Verification items for this drawing (mm, ordinates from the low corner). A direction names the side the tool comes from. Coordinates: 2 decimals unless noted, no trailing zeros. Write each loop counter-clockwise with the first axis right and the second up, starting at its lowest first coordinate (ties: lowest second). Pieces come first, ordered by that corner, then holes. Notation, with made-up numbers: (-35, 82.25) -> (14, 82.25) arc R19 ccw to (14, 119.25) -> close; hole circle Ø6 at (37, 82). An arc over 180 degrees is marked (long way). One line per item, written item: value. Start each with the question number.
1) Draft check along X on the marked faces 1, 2 and 3. Enter one of: +X half, -X half, draft (parallel to the pull), parting line (faces both ways), or undercut.
2) Scan lines: line 1 along Y through (x, z) = (3.5, 17.25); line 2 along Z through (x, y) = (5.25, 0.55); line 3 along Y through (x, z) = (2.5, 17.5). Record each from-to range of solid material in increasing order. Write a range as [from, to].
3) Sectioned sample at C-C on y = 0.5. Enter the section's corners in (x, z) (1 decimal), plus the area to 3 significant figures.
4) Sectioned sample at A-A on x = 5.5. Enter the section's corners in (y, z), plus the area to 3 significant figures.
5) Set-up check for the marked faces 4 and 5: record each of +Z, -Z, +X, -X, +Y, -Y from which the full face is reachable in a straight line by a thin tool's end or side.
6) Gauge pin test, flat ends, axial feed: P1, Ø3, axis at x = 4.5, y = 4.5, coming from the -Z side; P2, Ø1, axis at y = 4, z = 16, coming from the -X side; P3, Ø1.5, axis at y = 1.5, z = 15.5, coming from the -X side. Record the tip position at first contact, or that the pin passes through.
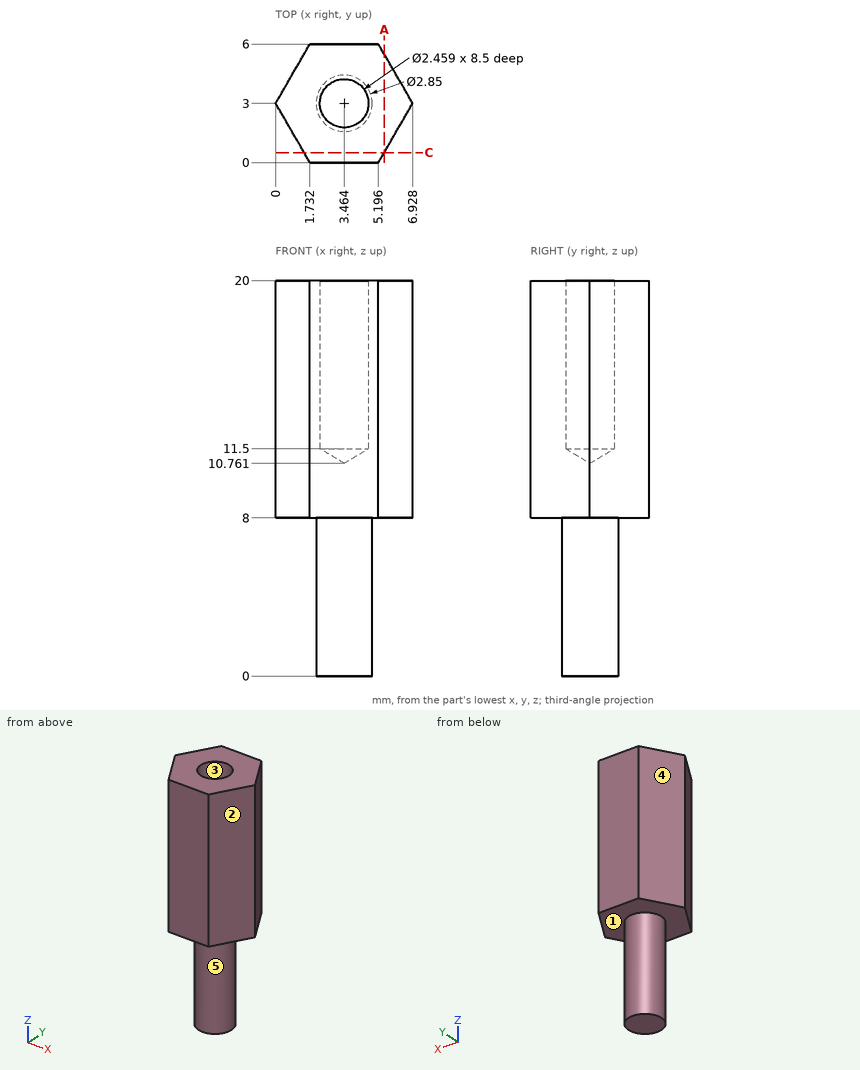
Answers:
1. face 1: draft
1. face 2: +X half
1. face 3: undercut
2. line 1: y = [0, 1.77], [4.23, 6]
2. line 2: z = [8, 20]
2. line 3: y = [0, 2.24], [3.76, 6]
3. outline: (1.4, 8) -> (5.5, 8) -> (5.5, 20) -> (1.4, 20) -> close
3. area: 48.5 mm2
4. outline: (0.53, 8) -> (5.47, 8) -> (5.47, 20) -> (0.53, 20) -> close
4. area: 59.4 mm2
5. face 4: +Z, -Z, -X, +Y
5. face 5: -Z
6. P1: stops at z = 0
6. P2: stops at x = 0.29
6. P3: stops at x = 0.43
